Work out the finished part from the listing and answer in its coordinate system (mm). A direction names the side the tool comes from. Coordinates: 2 decimals unless noted, no trailing zeros. Write each loop counter-clockwise with the first axis right and the second up, starting at its lowest first coordinate (ties: lowest second). Pieces come first, ordered by that corner, then holes. Notation, with made-up numbers: (33.25, -0.5) - (73.25, -0.5) arc R9 cw to (73.25, 8.5) - close; hole circle Ø2 at (-8.75, 31.5). An arc over 180 degrees is marked (long way). Use a Markdown table: item, result. Add a question column.
(1) Given pin 1 Ø8 at (x, y) = (-1, -1.5) entering from +Z; pin 2 Ø2 at (x, y) = (-5.5, 5) entering from +Z; pin 3 Ø1 at (x, y) = (13.5, -11) entering from -Z, each flat-ended and moving along its own axis, determine where each tip first touches the part or whether it passes through.
(2) Find the intervals of material crossed by line 1 (Y direction, x = 0, z = 5.8); line 2 (Y direction, x = -8.5, z = 3.5); line 3 (X direction, y = 12, z = 5), in increasing order. Write a range as from..to.
(3) The part is cut by section C-C, the plane z = 5.5. Give the vertices of the cut face in (x, y), then the cut area to 3 significant figures.
(4) The part is cut by section D-D, the plane z = -0.5. Give the vertices of the cut face in (x, y) (3 decimals), then the cut area to 3 significant figures.
(5) A tool of negligible diameter and unlimited length cuts with its end or side. For faces 1 (the face through (-12, -11, 7)), 2 (the face through (0.1, -3.3, 2)), 3 (the face through (1.08, -4.88, -1.97)), from which of +Z, -Z, +X, -X, +Y, -Y can it reach the whole face along a straight path? Write none if from no direction.
(6) For a pull along X with two mould halves and no side action, classify faces 4 (the face through (1.08, -4.88, 1.51)), 5 (the face through (-0.1, 11.3, 7)), 6 (the face through (-3.496, -15.742, 0.125)), 7 (the face through (-3.47, -15.62, 4.46)) as released by +X, released by -X, zero draft, split by the parting line, or undercut.
from build123d import *

# Parameters (mm, degrees)
ESQUISSE1_R             = 18
ESQUISSE1_R_2           = 16
BOSS_EXTRU_1_DEPTH      = 7
ESQUISSE1_R_3           = 13.75
ESQUISSE1_R_4           = 11
BOSS_EXTRU_1_2_DEPTH    = 7
ESQUISSE1_3_R           = 16
ESQUISSE1_3_R_2         = 13.75
BOSS_EXTRU_2_DEPTH      = 2
CHANFREIN1_SIZE         = 2
BOSS_EXTRU_3_DEPTH      = 4
BOSS_EXTRU_3_DEPTH_BACK = 2
ESQUISSE3_R             = 5
ESQUISSE3_R_2           = 3.125
ESQUISSE4_R             = 11
ESQUISSE4_R_2           = 3.834531167
BOSS_EXTRU_4_DEPTH      = 1


with BuildPart() as part:
    # Esquisse1 → Boss.-Extru.1 (new body)
    with BuildSketch(Plane.XY):
        Circle(ESQUISSE1_R)
        Circle(ESQUISSE1_R_2, mode=Mode.SUBTRACT)
    extrude(amount=BOSS_EXTRU_1_DEPTH)



with BuildPart() as body_2:
    # Esquisse1 → Boss.-Extru.1 2 (new body)
    with BuildSketch(Plane.XY):
        Circle(ESQUISSE1_R_3)
        Circle(ESQUISSE1_R_4, mode=Mode.SUBTRACT)
    extrude(amount=BOSS_EXTRU_1_2_DEPTH)


with BuildPart() as part_1:
    add(part.part)

    add(body_2.part)  # Boss.-Extru.2 merges body 2
    # Esquisse1_3 → Boss.-Extru.2 (add)
    with BuildSketch(Plane.XY):
        Circle(ESQUISSE1_3_R)
        Circle(ESQUISSE1_3_R_2, mode=Mode.SUBTRACT)
    extrude(amount=BOSS_EXTRU_2_DEPTH)

    # Chanfrein1
    chanfrein1_edges = [part_1.edges().sort_by_distance(p)[0] for p in [
        (-18, 0, 0),
    ]]
    chamfer(chanfrein1_edges, length=CHANFREIN1_SIZE)



with BuildPart() as body_2_2:
    # Esquisse3 → Boss.-Extru.3 (new, two sides: drawn at the far end of the back side and taken through both)
    with BuildSketch(Plane(origin=(0, 0, 0), x_dir=(-1, 0, 0), z_dir=(0, 0, -1)).offset(-BOSS_EXTRU_3_DEPTH_BACK)):
        Circle(ESQUISSE3_R)
        Circle(ESQUISSE3_R_2, mode=Mode.SUBTRACT)
    extrude(amount=BOSS_EXTRU_3_DEPTH + BOSS_EXTRU_3_DEPTH_BACK)


with BuildPart() as part_2:
    add(part_1.part)

    add(body_2_2.part)  # Boss.-Extru.4 merges body 2 2
    # Esquisse4 → Boss.-Extru.4 (add)
    with BuildSketch(Plane(origin=(0, 0, 0), x_dir=(-1, 0, 0), z_dir=(0, 0, -1))):
        Circle(ESQUISSE4_R)
        Circle(ESQUISSE4_R_2, mode=Mode.SUBTRACT)
    extrude(amount=-BOSS_EXTRU_4_DEPTH)


solid = part_2.part
Model answer:
| question | item | result |
|---|---|---|
| 1 | pin 1 | z = 2 |
| 1 | pin 2 | z = 1 |
| 1 | pin 3 | z = 0.91 |
| 2 | line 1 | -18..-16, -13.75..-11, 11..13.75, 16..18 |
| 2 | line 2 | -15.87..-13.56, -10.81..-6.98, 6.98..10.81, 13.56..15.87 |
| 2 | line 3 | -13.42..-10.58, -6.71..6.71, 10.58..13.42 |
| 3 | outline | circle Ø36 at (0, 0); circle Ø27.5 at (0, 0); hole circle Ø32 at (0, 0); hole circle Ø22 at (0, 0) |
| 3 | area | 427 mm^2 |
| 4 | outline | circle Ø10 at (0, 0); hole circle Ø6.25 at (0, 0) |
| 4 | area | 47.9 mm^2 |
| 5 | face 1 | +Z, +X, -X, +Y, -Y |
| 5 | face 2 | +Z |
| 5 | face 3 | -Z |
| 6 | face 4 | undercut |
| 6 | face 5 | zero draft |
| 6 | face 6 | split by the parting line |
| 6 | face 7 | undercut |
